Can you work these out from the model? Positions are in its coordinate system, mm. A direction names the side the tool comes from. Give positions to 0.01 mm unless a question says otherwise; leave off trailing zeros. Order: outer loops, then holes, each group sorted by start corner. A loop starts at its lowest first (then second) coordinate and runs counter-clockwise, first axis right, second up.
```python
from build123d import *

# Parameters (mm, degrees)
SKETCH1_R           = 20
SKETCH1_R_2         = 10
SKETCH1_R_3         = 2.1
BOSS_EXTRUDE1_DEPTH = 5
CUT_EXTRUDE1_DEPTH  = 6
FILLET1_R           = 1


with BuildPart() as part:
    # Sketch1 → Boss-Extrude1 (new body)
    with BuildSketch(Plane(origin=(0, 0, 0), x_dir=(1, 0, 0), z_dir=(0, 1, 0))):
        Circle(SKETCH1_R)
        Circle(SKETCH1_R_2, mode=Mode.SUBTRACT)
        with Locations((0, 15.25)):
            Circle(SKETCH1_R_3, mode=Mode.SUBTRACT)
        with Locations((13.206887408, -7.625)):
            Circle(SKETCH1_R_3, mode=Mode.SUBTRACT)
        with Locations((-13.206887408, -7.625)):
            Circle(SKETCH1_R_3, mode=Mode.SUBTRACT)
    extrude(amount=BOSS_EXTRUDE1_DEPTH)

    # Sketch2 → Cut-Extrude1 (cut, through all)
    with BuildSketch(Plane(origin=(0, 5, 0), x_dir=(1, 0, 0), z_dir=(0, 1, 0))):
        with BuildLine():
            ThreePointArc((-5.028195952, 14.397213115), (0, 10.15), (5.028195952, 14.397213115))
            ThreePointArc((5.028195952, 14.397213115), (13.206887408, 7.625), (14.982450277, -2.844061128))
            ThreePointArc((14.982450277, -2.844061128), (8.790157848, -5.075), (9.954254325, -11.553151987))
            ThreePointArc((9.954254325, -11.553151987), (0, -15.25), (-9.954254325, -11.553151987))
            ThreePointArc((-9.954254325, -11.553151987), (-8.790157848, -5.075), (-14.982450277, -2.844061128))
            ThreePointArc((-14.982450277, -2.844061128), (-13.206887408, 7.625), (-5.028195952, 14.397213115))
        make_face()
    extrude(amount=-CUT_EXTRUDE1_DEPTH, mode=Mode.SUBTRACT)

    # Fillet1
    fillet1_edges = [part.edges().sort_by_distance(p)[0] for p in [
        (-14.982450277, 2.5, 2.844061128),
        (-5.028195952, 2.5, -14.397213115),
        (5.028195952, 2.5, -14.397213115),
        (14.982450277, 2.5, 2.844061128),
        (9.954254325, 2.5, 11.553151987),
        (-9.954254325, 2.5, 11.553151987),
    ]]
    fillet(fillet1_edges, radius=FILLET1_R)


solid = part.part
```
1) Suppose I cut it at C-C (x = -12). Please give me the cut outline in (y, z), and give its area (3 significant figures).
2) I'm going to push flat-ended pins straight in: pin 1 Ø1 at (y, z) = (2, 7) entering from +X; pin 2 Ø3 at (y, z) = (3.5, 9.5) entering from +X. Where does each tip first touch, or does it pass through?
3) Which directions (+Z, -Z, +X, -X, +Y, -Y) give clear straight access to the entire face, cutting with the end or side of a thin tool? Please do faces 1 (the face through (8.834, 2.535, 5.001)), 2 (the face through (9, 5, 9)).
4) Suppose I cut it at A-A (x = 0). Please give me the cut outline in (y, z), and give its area (3 significant figures).
5) We'd pull the mould along Z, two halves only. Please class faces 3 (the face through (-4.336, 2.465, 19.524)), 4 (the face through (-14.755, 2.465, 6.206)), 5 (the face through (9, 0, 9)): +Z half, -Z half, draft (parallel to the pull), parting line (faces both ways), or undercut.
6) If I drill on line 1 (Z direction, x = 0, y = 2.95); line 2 (Z direction, x = -13, y = 4.5); line 3 (X direction, y = 2.6, z = 9), over which ranges is the centre line in solid material (lowest first)?
7) Suppose I cut it at B-B (z = 0). Please give me the cut outline in (x, y).
8) Suppose I cut it at D-D (z = -8). Please give me the cut outline in (x, y), and give its area (3 significant figures).
Results:
1. outline: (0, -16) - (5, -16) - (5, -9.41) - (0, -9.41) - close; (0, 2.67) - (5, 2.67) - (5, 5.91) - (0, 5.91) - close; (0, 9.34) - (5, 9.34) - (5, 16) - (0, 16) - close
1. area: 82.4 mm2
2. pin 1: stops at x = 18.91
2. pin 2: stops at x = 18.33
3. face 1: +Y, -Y
3. face 2: +Z, -Z, +X, -X, +Y
4. outline: (0, -20) - (5, -20) - (5, -17.35) - (0, -17.35) - close; (0, -13.15) - (5, -13.15) - (5, -10.15) - (0, -10.15) - close; (0, 15.25) - (5, 15.25) - (5, 20) - (0, 20) - close
4. area: 52.0 mm2
5. face 3: parting line
5. face 4: undercut
5. face 5: draft
6. line 1: z = -20 to -17.35, -13.15 to -10.15, 15.25 to 20
6. line 2: z = -15.2 to -7.97, 2.53 to 5.54, 9.71 to 15.2
6. line 3: x = -17.86 to -14.79, -11.62 to -8.3, 8.3 to 11.62, 14.79 to 17.86
7. outline: (-20, 0) - (-15.25, 0) - (-15.25, 5) - (-20, 5) - close; (15.25, 0) - (20, 0) - (20, 5) - (15.25, 5) - close
8. outline: (-18.33, 0) - (-12.98, 0) - (-12.98, 5) - (-18.33, 5) - close; (12.98, 0) - (18.33, 0) - (18.33, 5) - (12.98, 5) - close
8. area: 53.5 mm2
